```python
from build123d import *

# Parameters (mm, degrees)
SKETCH2_W           = 20
SKETCH2_H           = 40
BOSS_EXTRUDE1_DEPTH = 0.5
SKETCH4_W           = 18
SKETCH4_H           = 38
BOSS_EXTRUDE2_DEPTH = 0.5
FILLET1_R           = 0.5


with BuildPart() as part:
    # Sketch2 → Boss-Extrude1 (new body)
    with BuildSketch(Plane.XY):
        Rectangle(SKETCH2_W, SKETCH2_H)
    extrude(amount=BOSS_EXTRUDE1_DEPTH)

    # Sketch4 → Boss-Extrude2 (add)
    with BuildSketch(Plane(origin=(0, 0, 0), x_dir=(-1, 0, 0), z_dir=(0, 0, -1))):
        Rectangle(SKETCH4_W, SKETCH4_H)
    extrude(amount=BOSS_EXTRUDE2_DEPTH)

    # Fillet1
    fillet1_edges = [part.edges().sort_by_distance(p)[0] for p in [
        (10, -20, 0.25),
        (-10, -20, 0.25),
        (-10, 20, 0.25),
        (10, 20, 0.25),
    ]]
    fillet(fillet1_edges, radius=FILLET1_R)


solid = part.part
```
Read the model definition and answer for the solid it produces. Units are mm, in the model's axes. Give positions to 0.01 mm unless a question says otherwise; leave off trailing zeros. Order: outer loops, then holes, each group sorted by start corner. A loop starts at its lowest first (then second) coordinate and runs counter-clockwise, first axis right, second up.
(1) Find section A-A (x = -1.75). Give the vertices of the cut face in (y, z), plus the area to 3 significant figures.
(2) Straight lines are drawn through the part: L1, parallel to Y at x = 8.5, z = -0.1; L2, parallel to X at y = 1, z = -0.1. For each, find the intervals that lie inside material, in ascending order.
(3) Find section C-C (z = -0.25). Give the vertices of the cut face in (x, y).
(4) Find section B-B (y = 10). Give the vertices of the cut face in (x, z), plus the area to 3 significant figures.
Result sheet:
1. outline: (-20, 0) - (-19, 0) - (-19, -0.5) - (19, -0.5) - (19, 0) - (20, 0) - (20, 0.5) - (-20, 0.5) - close
1. area: 39.0 mm2
2. L1: y = -19 to 19
2. L2: x = -9 to 9
3. outline: (-9, -19) - (9, -19) - (9, 19) - (-9, 19) - close
4. outline: (-10, 0) - (-9, 0) - (-9, -0.5) - (9, -0.5) - (9, 0) - (10, 0) - (10, 0.5) - (-10, 0.5) - close
4. area: 19.0 mm2
